Build history of the part. All positions in model axes, mm. A direction names the side the tool comes from. Give positions to 0.01 mm unless a question says otherwise; leave off trailing zeros. Loops run counter-clockwise (first coordinate to the right, second up) from the corner with the lowest first, then second, coordinate; pieces in that order, holes last.
1) 3-axis set-ups, long thin cutter, end or side, ignore diameter. For faces 1 (the flat face through (11, 69.086, 39)), 2 (the flat face through (-486.42, -63, 39)): which of +Z, -Z, +X, -X, +Y, -Y reach the whole face in a straight line?
2) Two-plate mould, pull along X, no slides. Class faces 3 (the flat face through (493.58, -63, 39)), 4 (the flat face through (503.58, -58, 39)), 5 (the flat face through (38, 65, 0)), 6 (the flat face through (-3, 59.086, 39)): +X half, -X half, draft (parallel to the pull), parting line (faces both ways), or undercut.
3) Flat gauge pins, fed straight in: P1, Ø2.5, axis at x = 499, y = 63, coming from the -Z side; P2, Ø4, axis at x = -269.5, y = 63, coming from the -Z side; P3, Ø8, axis at x = 255.5, z = 28, coming from the -Y side. Where does each tip first touch, or does it go through?
4) Band-saw the part on B-B on z = 12.5. State how many separate pieces and enclosed holes the cut face has, then the cut area to 3 significant figures.
5) Band-saw the part on A-A on y = -130. List the corners of the cut face in (x, z).
6) Wall check: line 1 (X direction, y = -0.5, z = 60); line 2 (Y direction, x = 0, z = 15); line 3 (Y direction, x = 437.5, z = 43.5). Give the ranges that are in metal, low to high.
7) Band-saw the part on C-C on x = 439.5. List the corners of the cut face in (y, z), then the cut area to 3 significant figures.
```python
from build123d import *

# Parameters (mm, degrees)
F0_W     = 10
F0_H     = 10
F0_W_2   = 980
F0_H_2   = 240
F1_DEPTH = 80
F2_R     = 2.5
F3_DEPTH = 30


with BuildPart() as f1:
    # F0 (on Top) → F1 (new body)
    with BuildSketch(Plane.XY):
        with Locations((-491.420456, 64.085509)):
            Rectangle(F0_W, F0_H)
        with Locations((3.579544, 64.085509)):
            Rectangle(F0_W_2, F0_H)
        with Locations((-491.420456, -60.914491)):
            Rectangle(F0_W, F0_H_2)
        with Locations((498.579544, 64.085509)):
            Rectangle(F0_W, F0_H)
        with Locations((498.579544, -60.914491)):
            Rectangle(F0_W, F0_H_2)
    extrude(amount=F1_DEPTH)

    # F2 (on face) → F3 (cut)
    with BuildSketch(Plane(origin=(0, 0, 0), x_dir=(1, 0, 0), z_dir=(0, 0, -1))):
        with Locations((-491.420456, 153.839529)):
            Circle(F2_R)
        with Locations((-491.420456, 52.106358)):
            Circle(F2_R)
        with Locations((-491.420456, -64.085509)):
            Circle(F2_R)
        with Locations((-269.96702, -64.085509)):
            Circle(F2_R)
        with Locations((0, -64.085509)):
            Circle(F2_R)
        with Locations((269.96702, -64.085509)):
            Circle(F2_R)
        with Locations((498.579544, -64.085509)):
            Circle(F2_R)
        with Locations((498.579544, 52.106358)):
            Circle(F2_R)
        with Locations((498.579544, 153.839529)):
            Circle(F2_R)
    extrude(amount=-F3_DEPTH, mode=Mode.SUBTRACT)


solid = f1.part
```
Findings below:
1. face 1: +Z, -Z, +X, -X, +Y
1. face 2: +Z, -Z, -Y
2. face 3: undercut
2. face 4: +X half
2. face 5: draft
2. face 6: undercut
3. P1: stops at z = 30
3. P2: stops at z = 0
3. P3: stops at y = 59.09
4. separate pieces: 1
4. enclosed holes: 9
4. area: 14,600 mm2
5. outline: (-496.42, 0) - (-486.42, 0) - (-486.42, 80) - (-496.42, 80) - close; (493.58, 0) - (503.58, 0) - (503.58, 80) - (493.58, 80) - close
6. line 1: x = -496.42 to -486.42, 493.58 to 503.58
6. line 2: y = 59.09 to 61.59, 66.59 to 69.09
6. line 3: y = 59.09 to 69.09
7. outline: (59.09, 0) - (69.09, 0) - (69.09, 80) - (59.09, 80) - close
7. area: 800 mm2
